Job drawing, mm, ordinate dimensions from the low corner. One solid piece. Give positions to 0.01 mm unless a question says otherwise; leave off trailing zeros. Loops run counter-clockwise (first coordinate to the right, second up) from the corner with the lowest first, then second, coordinate; pieces in that order, holes last. Notation, with made-up numbers: (60, -27.75) - (74, -27.75) arc R10 cw to (74, -17.75) - close; hole circle Ø9 at (-4.75, 45). An arc over 180 degrees is marked (long way). Answer as CSV lines item,"result". Start each with the question number.
Item 1: Saw through at B-B on y = 5. Give the cut face in (x, z), plus the area to 3 significant figures.
Item 2: Pin check, flat tips, straight feed: pin 1 (5 mm diameter, centred on x = 5, y = 5, fed in from +Z); pin 2 (1.5 mm diameter, centred on x = 4, y = 12, fed in from +Z). Stop position of each tip, or through.
Item 3: Saw through at D-D on z = 1.65. Give the cut face in (x, y).
Item 4: Pull direction Y, two halves, no side cores. Call the marked faces 1, 2 and 3: pulls with the +Y half, pulls with the -Y half, needs draft (parallel to the pull), parting line crosses it, or undercut.
Item 5: Drill centre lines: L1, parallel to X at y = 3.25, z = 0.7; L2, parallel to X at y = 21, z = 2.85; L3, parallel to Y at x = 5.75, z = 0.65. Where is each one in solid material? Low to high. Write a range as from..to.
Item 6: Saw through at A-A on z = 4.85. Give the cut face in (x, y), plus the area to 3 significant figures.
Item 7: Saw through at C-C on x = 5. Give the cut face in (y, z), plus the area to 3 significant figures.
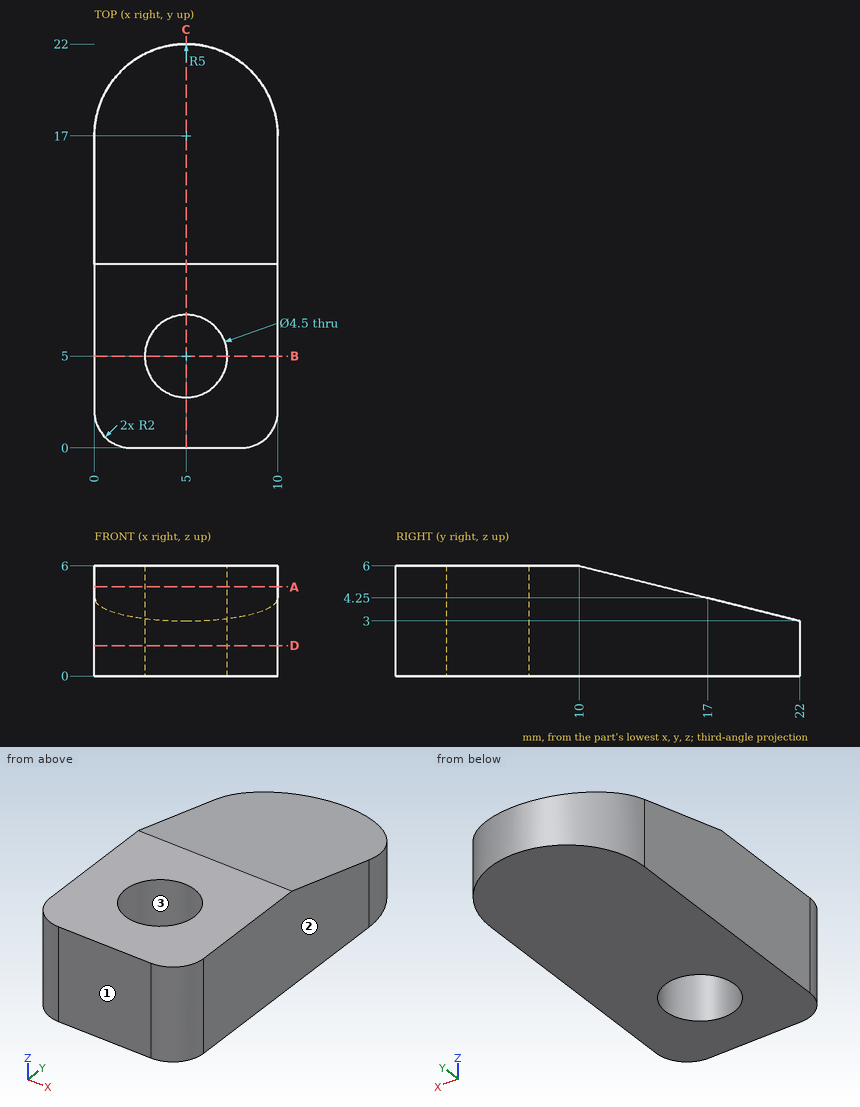
Responses:
1,outline,"(0, 0) - (2.75, 0) - (2.75, 6) - (0, 6) - close; (7.25, 0) - (10, 0) - (10, 6) - (7.25, 6) - close"
1,area,"33.0 mm2"
2,pin 1,"z = 6"
2,pin 2,"z = 5.69"
3,outline,"(0, 2) arc R2 ccw to (2, 0) - (8, 0) arc R2 ccw to (10, 2) - (10, 17) arc R5 ccw to (0, 17) - close; hole circle Ø4.5 at (5, 5)"
4,face 1,"pulls with the -Y half"
4,face 2,"needs draft"
4,face 3,"undercut"
5,L1,"0..3.59, 6.41..10"
5,L2,"2..8"
5,L3,"0..2.88, 7.12..21.94"
6,outline,"(0, 2) arc R2 ccw to (2, 0) - (8, 0) arc R2 ccw to (10, 2) - (10, 14.6) - (0, 14.6) - close; hole circle Ø4.5 at (5, 5)"
6,area,"128 mm2"
7,outline,"(0, 0) - (2.75, 0) - (2.75, 6) - (0, 6) - close; (7.25, 0) - (22, 0) - (22, 3) - (10, 6) - (7.25, 6) - close"
7,area,"87.0 mm2"
